Geometry check sheet. Reference: the model listing, model coordinates, mm. Face numbers are marked on the shaded views. A direction names the side the tool comes from. Give positions to 0.01 mm unless a question says otherwise; leave off trailing zeros. Order: outer loops, then holes, each group sorted by start corner. A loop starts at its lowest first (then second) coordinate and runs counter-clockwise, first axis right, second up. Notation, with made-up numbers: M -4.5,-14.75 L 46.5,-14.75 A16 ccw 46.5,-10.75 Z; hole C 74,79 d5. An arc over 180 degrees is marked long. Answer as CSV lines item,"result".
from build123d import *

# Parameters (mm, degrees)
SKETCH_1_R          = 8
EXTRUDE_1_DEPTH     = 2.5
SKETCH_4_R          = 9
EXTRUDE_2_DEPTH     = 1.1
SKETCH_2_R          = 4
CUT_EXTRUDE_1_DEPTH = 6
SKETCH_3_R          = 6.8
SKETCH_3_R_2        = 5
CUT_EXTRUDE_2_DEPTH = 0.2


with BuildPart() as part:
    # 草圖1 → 填料-伸長1 (new body, symmetric)
    with BuildSketch(Plane.XY):
        Circle(SKETCH_1_R)
    extrude(amount=EXTRUDE_1_DEPTH, both=True)

    # 草圖4 → 填料-伸長2 (add)
    with BuildSketch(Plane(origin=(0, 0, -2.5), x_dir=(-1, 0, 0), z_dir=(0, 0, -1))):
        Circle(SKETCH_4_R)
    extrude(amount=-EXTRUDE_2_DEPTH)

    # 草圖2 → 除料-伸長1 (cut, through all)
    with BuildSketch(Plane.XY.offset(2.5)):
        Circle(SKETCH_2_R)
    extrude(amount=-CUT_EXTRUDE_1_DEPTH, mode=Mode.SUBTRACT)

    # 草圖3 → 除料-伸長2 (cut)
    with BuildSketch(Plane.XY.offset(2.5)):
        Circle(SKETCH_3_R)
        Circle(SKETCH_3_R_2, mode=Mode.SUBTRACT)
    cut_extrude_2 = extrude(amount=-CUT_EXTRUDE_2_DEPTH, mode=Mode.SUBTRACT)

    # 鏡射1: 除料-伸長2 across plane
    add(cut_extrude_2.mirror(Plane.XY), mode=Mode.SUBTRACT)


solid = part.part
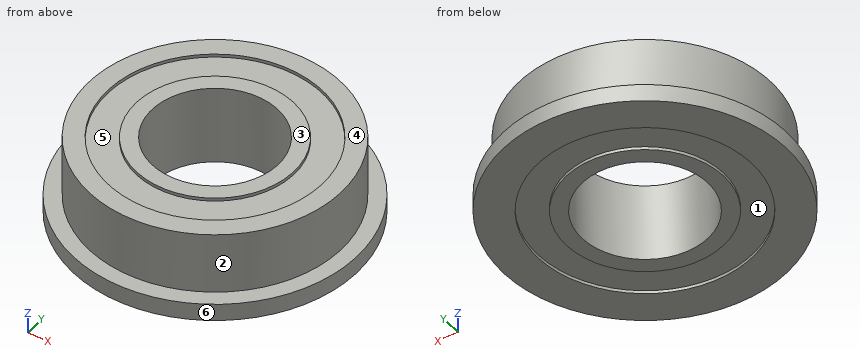
(1) Section check A-A on y = 0. Enter the section's corners in (x, z), then the cut area to 3 significant figures.
The answers:
outline,"M -9,-2.5 L -6.8,-2.5 L -6.8,-2.3 L -5,-2.3 L -5,-2.5 L -4,-2.5 L -4,2.5 L -5,2.5 L -5,2.3 L -6.8,2.3 L -6.8,2.5 L -8,2.5 L -8,-1.4 L -9,-1.4 Z; M 4,-2.5 L 5,-2.5 L 5,-2.3 L 6.8,-2.3 L 6.8,-2.5 L 9,-2.5 L 9,-1.4 L 8,-1.4 L 8,2.5 L 6.8,2.5 L 6.8,2.3 L 5,2.3 L 5,2.5 L 4,2.5 Z"
area,"40.8 mm2"
(2) Gauge pin test, flat ends, axial feed: P1, Ø2, axis at y = -3, z = -1.5, coming from the -X side; P2, Ø1.5, axis at y = -0.5, z = 1, coming from the +X side. Record the tip position at first contact, or that the pin passes through.
The answers:
P1,"stops at x = -8.77"
P2,"stops at x = 8"
(3) Material ranges on line 1 (Y direction, x = 0, z = -2.35); line 2 (Y direction, x = 0, z = 2.4); line 3 (Y direction, x = 0, z = -0.05), recorded low to high.
The answers:
line 1,"y = -9 to -6.8, -5 to -4, 4 to 5, 6.8 to 9"
line 2,"y = -8 to -6.8, -5 to -4, 4 to 5, 6.8 to 8"
line 3,"y = -8 to -4, 4 to 8"
(4) Section check D-D on x = -6. Enter the section's corners in (y, z), then the cut area to 3 significant figures.
The answers:
outline,"M -6.71,-2.5 L -3.2,-2.5 L -3.2,-2.3 L 3.2,-2.3 L 3.2,-2.5 L 6.71,-2.5 L 6.71,-1.4 L 5.29,-1.4 L 5.29,2.5 L 3.2,2.5 L 3.2,2.3 L -3.2,2.3 L -3.2,2.5 L -5.29,2.5 L -5.29,-1.4 L -6.71,-1.4 Z"
area,"53.5 mm2"
(5) Section check C-C on z = 0. Enter the section's corners in (x, y), then the cut area to 3 significant figures.
The answers:
outline,"C 0,0 d16; hole C 0,0 d8"
area,"151 mm2"
(6) Draft check along X on the marked faces 4, 5 and 6. Enter one of: +X half, -X half, draft (parallel to the pull), parting line (faces both ways), or undercut.
The answers:
face 4,"draft"
face 5,"undercut"
face 6,"parting line"
(7) Tool access check on the marked faces 1, 2 and 3. Record the directions out of +Z, -Z, +X, -X, +Y, -Y that give a thin tool (end or side, any length) a straight path to the whole face; none if there is none.
The answers:
face 1,"-Z"
face 2,"+Z"
face 3,"+Z, +X, -X, +Y, -Y"
